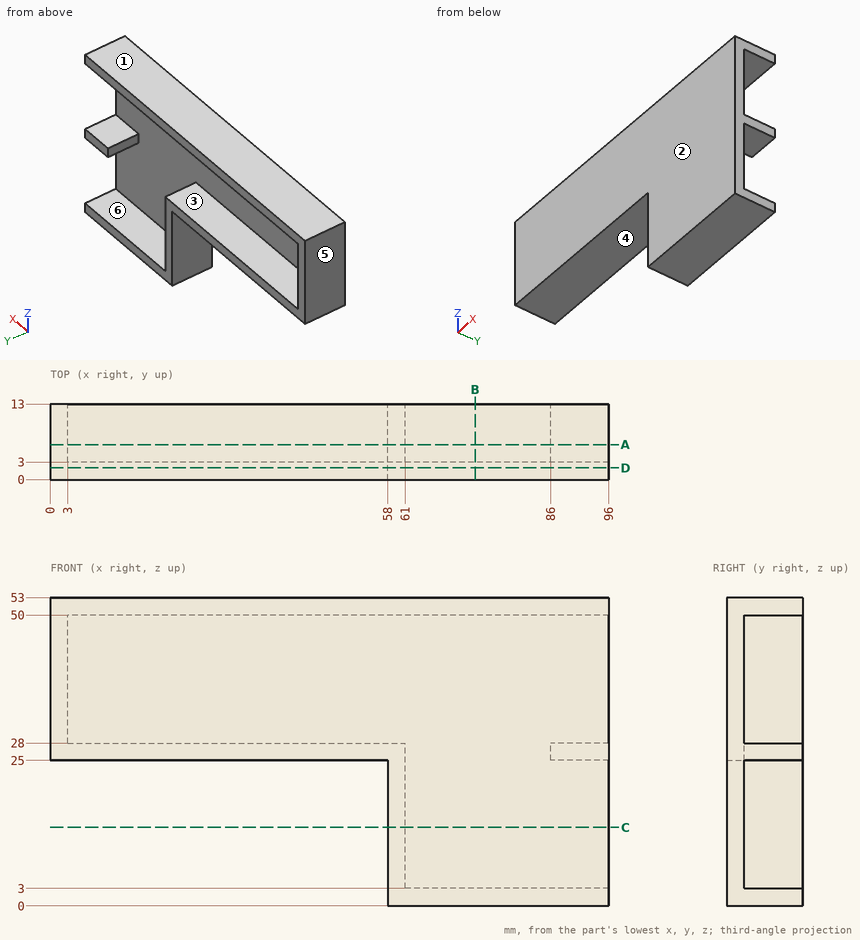
Print and shaded views of the part. All mm, measured from the part's lowest x, y and z. A direction names the side the tool comes from. Give positions to 0.01 mm unless a question says otherwise; leave off trailing zeros. Write each loop counter-clockwise with the first axis right and the second up, starting at its lowest first coordinate (ties: lowest second). Pieces come first, ordered by that corner, then holes. Notation, with made-up numbers: M -19.75,82.5 L 6.25,82.5 A19 ccw 6.25,88.5 Z; hole C -5.5,31.25 d7. An arc over 180 degrees is marked long. Use a Markdown table: item, result.
1) Cut at D-D (y = 2). List the corners of the cut face in (x, z).
Responses:
| item | result |
|---|---|
| outline | M 0,25 L 58,25 L 58,0 L 96,0 L 96,53 L 0,53 Z |
2) Cut at C-C (z = 13.5). List the corners of the cut face in (x, y).
Responses:
| item | result |
|---|---|
| outline | M 58,0 L 96,0 L 96,3 L 61,3 L 61,13 L 58,13 Z |
3) Cut at B-B (x = 73). List the corners of the cut face in (y, z), and give its area (3 significant figures).
Responses:
| item | result |
|---|---|
| outline | M 0,0 L 13,0 L 13,3 L 3,3 L 3,50 L 13,50 L 13,53 L 0,53 Z |
| area | 219 mm2 |
4) Drill centre lines: line 1 (Z direction, x = 86.5, y = 7); line 2 (Z direction, x = 28.5, y = 7.25); line 3 (Z direction, x = 81.5, y = 12). Where is each one in solid material? Low to high. Write a range as from..to.
Responses:
| item | result |
|---|---|
| line 1 | z = 0..3, 25..28, 50..53 |
| line 2 | z = 25..28, 50..53 |
| line 3 | z = 0..3, 50..53 |
5) Cut at A-A (y = 6). List the corners of the cut face in (x, z), and give its area (3 significant figures).
Responses:
| item | result |
|---|---|
| outline | M 0,25 L 58,25 L 58,0 L 96,0 L 96,3 L 61,3 L 61,28 L 3,28 L 3,50 L 96,50 L 96,53 L 0,53 Z; M 86,25 L 96,25 L 96,28 L 86,28 Z |
| area | 747 mm2 |
6) Tool access for the marked faces 4, 5 and 6: list every direction of +Z, -Z, +X, -X, +Y, -Y with a clear straight run to the whole face (end or side of a thin tool).
Responses:
| item | result |
|---|---|
| face 4 | -Z, -X, +Y, -Y |
| face 5 | +Z, -Z, -X, +Y, -Y |
| face 6 | +X, +Y |
7) Pull direction Z, two halves, no side cores. Call the marked faces 1, 2 and 3: +Z half, -Z half, draft (parallel to the pull), parting line (faces both ways), or undercut.
Responses:
| item | result |
|---|---|
| face 1 | +Z half |
| face 2 | draft |
| face 3 | undercut |
8) Pin check, flat tips, straight feed: pin 1 (6.5 mm diameter, centred on x = 43.5, y = 4.5, fed in from -Z); pin 2 (6 mm diameter, centred on x = 21, z = 30.5, fed in from +Y); pin 3 (5 mm diameter, centred on y = 6.5, z = 10, fed in from +X); pin 4 (3 mm diameter, centred on y = 9, z = 36.5, fed in from +X). Stop position of each tip, or through.
Responses:
| item | result |
|---|---|
| pin 1 | stops at z = 25 |
| pin 2 | stops at y = 13 |
| pin 3 | stops at x = 61 |
| pin 4 | stops at x = 3 |
